Part model, mm, in its own coordinate system. Face numbers are marked on the shaded views. A direction names the side the tool comes from. Coordinates: 2 decimals unless noted, no trailing zeros. Loops run counter-clockwise (first coordinate to the right, second up) from the corner with the lowest first, then second, coordinate; pieces in that order, holes last. Notation, with made-up numbers: M -15,53.5 L -9,53.5 A14 ccw -9,78.5 Z; hole C 68,11.5 d1. An arc over 180 degrees is marked long. Use a Markdown table: item, result. Add a question column.
1) Band-saw the part on A-A (z = 12.5). List the corners of the cut face in (x, y).
2) Wall check: probe 1 along X at (y, z) = (39.5, 9.25); probe 2 along Y at (x, z) = (6.5, -2.75). Give the ranges that are in metal, low to high. Write a range as from..to.
3) Tool access for the marked faces 4, 5, 6 and 7: list every direction of +Z, -Z, +X, -X, +Y, -Y with a clear straight run to the whole face (end or side of a thin tool).
4) Band-saw the part on B-B (z = 7). List the corners of the cut face in (x, y).
5) Pin check, flat tips, straight feed: pin 1 Ø1.5 at (x, z) = (16, 6) entering from +Y; pin 2 Ø1 at (x, y) = (5.5, 30.5) entering from -Z; pin 3 Ø11 at (x, z) = (4, 17) entering from -Y. Stop position of each tip, or through.
6) Pull direction Y, two halves, no side cores. Call the marked faces 1, 2 and 3: released by +Y, released by -Y, zero draft, split by the parting line, or undercut.
7) Band-saw the part on C-C (x = 43). List the corners of the cut face in (y, z), plus the area to 3 significant figures.
Autodesk Fusion 360 part; units mm, degrees
sketch "Sketch1" plane through (0, 0, 0) normal (0, 0, 1) x (1, 0, 0)
  line L0 (0, 40) -> (10, 40)
  line L1 (10, 40) -> (10, 10)
  line L2 (0, 0) -> (0, 40)
  line L3 (40, 0) -> (40, 10)
  line L4 (40, 10) -> (10, 10)
  line L5 (0, 10) -> (0, 0)
  line L6 (0, 0.1) -> (40, 0)
  dimension "d1" = 10
  dimension "d2" = 40
  dimension "d3" = 40
  dimension "d4" = 10
extrude "Extrude1" add sketch "Sketch1" along normal blind 10
sketch "Sketch2" plane through (40, 0, 0) normal (1, 0, 0) x (0, 1, 0)
  line L0 (0, 0) -> (10, 0)
  line L1 (10, 0) -> (10, 10)
  line L2 (10, 10) -> (0, 10)
  line L3 (0, 10) -> (0, 0)
  line L4 (0, 20) -> (10, 20)
  line L5 (10, 20) -> (10, -10)
  line L6 (10, -10) -> (0, -10)
  line L7 (0, -10) -> (0, 20)
  dimension "d7" = 10
  dimension "d8" = 30
extrude "Extrude2" add sketch "Sketch2" along normal blind 10
sketch "Sketch3" plane through (40, 0, 0) normal (-1, 0, 0) x (0, -1, 0)
  line L0 (-10, 10) -> (0, 10)
  line L1 (0, 10) -> (0, 20)
  line L2 (0, 20) -> (-10, 20)
  line L3 (-10, 20) -> (-10, 10)
extrude "Extrude3" cut sketch "Sketch3" against normal blind 6
move_face "OffsetFaces1" offset -6 1 faces at (40, 3.3333, -6.6667)
sketch "Sketch4" plane through (0, 40, 0) normal (0, 1, 0) x (-1, 0, 0)
  line L0 (-10, 0) -> (0, 0)
  line L1 (0, 0) -> (0, 10)
  line L2 (0, 10) -> (-10, 10)
  line L3 (-10, 10) -> (-10, 0)
  line L4 (-10, 20) -> (0, 20)
  line L5 (0, 20) -> (0, -10)
  line L6 (0, -10) -> (-10, -10)
  line L7 (-10, -10) -> (-10, 20)
extrude "Extrude4" add sketch "Sketch4" along normal blind 4
fillet "Fillet1" radius 8 1 edges at (0, 0.1, 5)
fillet "Fillet2" radius 8 1 edges at (10, 10, 5)
hole "Hole1" at (5.0001, 40, 14.9993) direction (0, 1, 0) diameter 3 end through all
hole "Hole2" at (5.0001, 40, -4.9998) direction (0, 1, 0) diameter 3 end through all
hole "Hole3" at (46, 5.0035, -5.0012) direction (1, 0, 0) diameter 3 end through all
hole "Hole4" at (46, 5.0005, 14.9997) direction (1, 0, 0) diameter 3 end through all
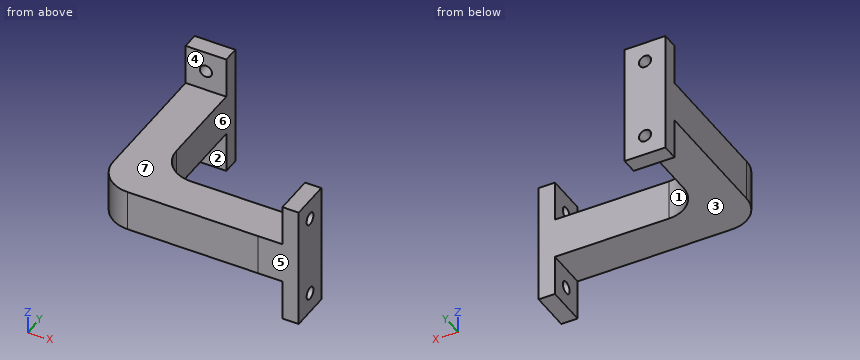
Entries:
| question | item | result |
|---|---|---|
| 1 | outline | M 0,40 L 10,40 L 10,44 L 0,44 Z; M 46,0 L 50,0 L 50,10 L 46,10 Z |
| 2 | probe 1 | 0..10 |
| 2 | probe 2 | 40..44 |
| 3 | face 4 | +Z, +X, -X, -Y |
| 3 | face 5 | +Z, -Z, +X, -X, -Y |
| 3 | face 6 | +Z, -Z, +X, +Y |
| 3 | face 7 | +Z, -X, -Y |
| 4 | outline | M 0,8.08 A8 ccw 7.98,0.08 L 40,0 L 50,0 L 50,10 L 18,10 A8 cw 10,18 L 10,44 L 0,44 Z |
| 5 | pin 1 | y = 10.49 |
| 5 | pin 2 | z = 0 |
| 5 | pin 3 | y = 40 |
| 6 | face 1 | released by +Y |
| 6 | face 2 | released by -Y |
| 6 | face 3 | zero draft |
| 7 | outline | M 0,0 L 10,0 L 10,10 L 0,10 Z |
| 7 | area | 100 mm2 |
